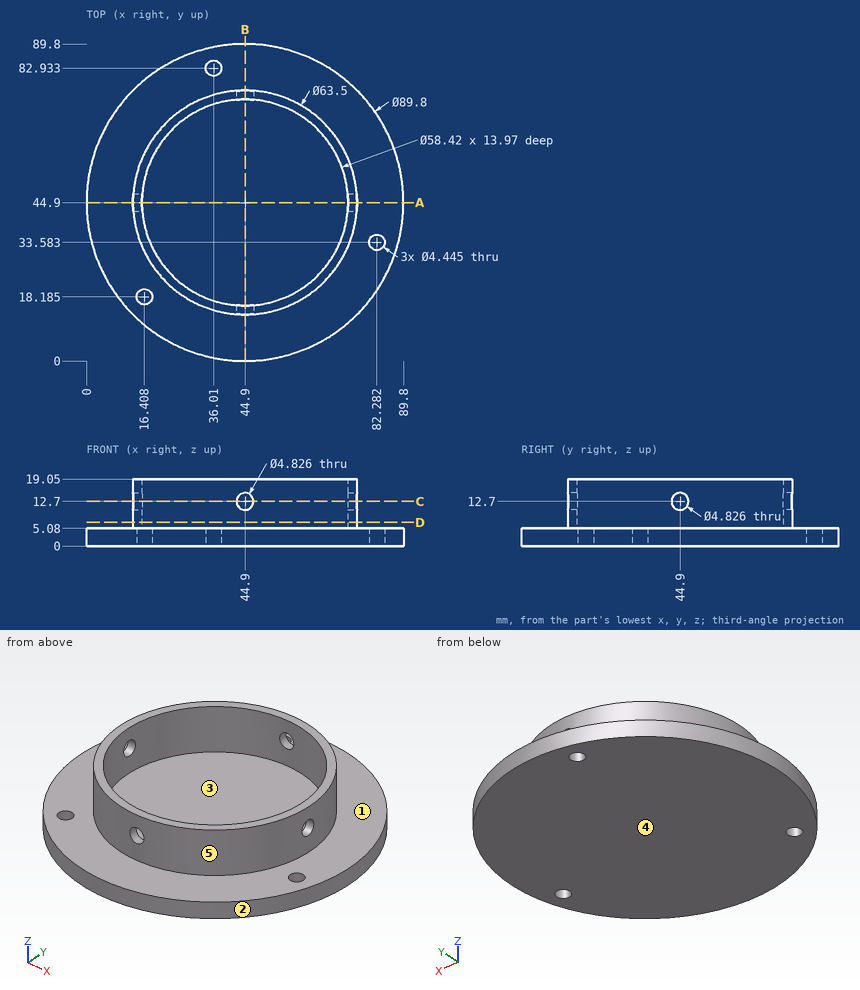
Could you check a few things on this drawing? It's one solid part, dimensions in mm from its lowest x, y, z. A direction names the side the tool comes from. Coordinates: 2 decimals unless noted, no trailing zeros. Loops run counter-clockwise (first coordinate to the right, second up) from the corner with the lowest first, then second, coordinate; pieces in that order, holes last.
1. Imagine slicing it at D-D (z = 6.75). Please give me the cut outline in (x, y).
2. For P1, Ø4, axis at y = 73.5, z = 15.5, coming from the -X side (1 decimal); P2, Ø3, axis at y = 33.5, z = 12, coming from the -X side; P3, Ø1.5, axis at x = 24, z = 14, coming from the -Y side (1 decimal); P4, Ø4, axis at y = 44.9, z = 12.7, coming from the +X side, each with a flat end and sliding along its axis, tell me the tip position at first contact or that it passes through.
3. For the marked faces 1 and 2, which set-ups out of +Z, -Z, +X, -X, +Y, -Y let a thin tool reach every point of the face, with its end or its side?
4. Imagine slicing it at C-C (z = 12.7). Please give me the cut outline in (x, y).
5. We'd pull the mould along X, two halves only. Please class the marked faces 3, 4 and 5: released by +X, released by -X, zero draft, split by the parting line, or undercut.
6. Imagine slicing it at A-A (y = 44.9). Please give me the cut outline in (x, z).
7. I need wall thicknesses on L1, parallel to X at y = 44.9, z = 8.25; L2, parallel to Z at x = 65, y = 51; L3, parallel to Z at x = 75, y = 44.9. Which ranges of each line are inside material? Lowest first, please.
Computed values:
1. outline: circle Ø63.5 at (44.9, 44.9); hole circle Ø58.42 at (44.9, 44.9)
2. P1: stops at x = 27.6
2. P2: stops at x = 14.73
2. P3: stops at y = 20.4
2. P4: passes through
3. face 1: +Z
3. face 2: +Z, -Z
4. outline: (13.24, 42.49) arc R31.75 ccw to (42.49, 13.24) - (42.49, 15.79) arc R29.21 cw to (15.79, 42.49) - close; (13.24, 47.31) - (15.79, 47.31) arc R29.21 cw to (42.49, 74.01) - (42.49, 76.56) arc R31.75 ccw to start; (47.31, 13.24) arc R31.75 ccw to (76.56, 42.49) - (74.01, 42.49) arc R29.21 cw to (47.31, 15.79) - close; (47.31, 74.01) arc R29.21 cw to (74.01, 47.31) - (76.56, 47.31) arc R31.75 ccw to (47.31, 76.56) - close
5. face 3: undercut
5. face 4: zero draft
5. face 5: split by the parting line
6. outline: (0, 0) - (89.8, 0) - (89.8, 5.08) - (76.65, 5.08) - (76.65, 10.29) - (74.11, 10.29) - (74.11, 5.08) - (15.69, 5.08) - (15.69, 10.29) - (13.15, 10.29) - (13.15, 5.08) - (0, 5.08) - close; (13.15, 15.11) - (15.69, 15.11) - (15.69, 19.05) - (13.15, 19.05) - close; (74.11, 15.11) - (76.65, 15.11) - (76.65, 19.05) - (74.11, 19.05) - close
7. L1: x = 13.15 to 15.69, 74.11 to 76.65
7. L2: z = 0 to 5.08
7. L3: z = 0 to 10.29, 15.11 to 19.05
